```python
from build123d import *

# Parameters (mm, degrees)
RESSALTO_EXTRUS_O1_DEPTH       = 1.9
CONVERTER_S_LIDO1_DEPTH        = 0.7
ARESTA_FLANGE1_STRIP_W         = 8
ARESTA_FLANGE1_STRIP_H         = 1.2
ARESTA_FLANGE1_STRIP_CUT_DEPTH = 532
ARESTA_FLANGE1_DEPTH           = 532
RESSALTO_EXTRUS_O2_DEPTH       = 1.6


# Read off the part's stored shape, not the designer's step: Converter-Sólido1
# Sheet-metal steps are written as plain solids
with BuildPart() as part:
    # Esboço1 → Ressalto-extrusão1 (new body)
    with BuildSketch(Plane.XY):
        with BuildLine():
            Line((-266, -25), (-266, 61))
            Line((-266, 61), (266, 61))
            Line((266, 61), (266, -25))
            Line((266, -25), (208, -25))
            ThreePointArc((208, -25), (199.514718626, -21.485281374), (196, -13))
            Line((196, -13), (196, 0))
            Line((196, 0), (-196, 0))
            Line((-196, 0), (-196, -13))
            ThreePointArc((-196, -13), (-199.514718626, -21.485281374), (-208, -25))
            Line((-208, -25), (-266, -25))
        make_face()
    extrude(amount=RESSALTO_EXTRUS_O1_DEPTH)

    # Converter-Sólido1 outline → Converter-Sólido1 (cut)
    with BuildSketch(Plane.XY):
        with BuildLine():
            Line((-266, -25), (-208, -25))
            ThreePointArc((-208, -25), (-199.514718626, -21.485281374), (-196, -13))
            Line((-196, -13), (-196, 0))
            Line((-196, 0), (196, 0))
            Line((196, 0), (196, -13))
            ThreePointArc((196, -13), (199.514718626, -21.485281374), (208, -25))
            Line((208, -25), (266, -25))
            Line((266, -25), (266, 61))
            Line((266, 61), (-266, 61))
            Line((-266, 61), (-266, -25))
        make_face()
    extrude(amount=CONVERTER_S_LIDO1_DEPTH, mode=Mode.SUBTRACT)

    # Aresta-Flange1 strip (across the edge) → Aresta-Flange1 strip cut (cut)
    with BuildSketch(Plane(origin=(-266, 61, 0.7), x_dir=(0, -1, 0), z_dir=(1, 0, 0))):
        with Locations((-1.2, -0.6)):
            Rectangle(ARESTA_FLANGE1_STRIP_W, ARESTA_FLANGE1_STRIP_H)
    extrude(amount=ARESTA_FLANGE1_STRIP_CUT_DEPTH, mode=Mode.SUBTRACT)

    # Aresta-Flange1 section (across the edge) → Aresta-Flange1 (add)
    with BuildSketch(Plane(origin=(-266, 61, 0.7), x_dir=(0, -1, 0), z_dir=(1, 0, 0))):
        with BuildLine():
            Line((0, 1.6), (0, 24.2))
            Line((0, 24.2), (1.2, 24.2))
            Line((1.2, 24.2), (1.2, 1.6))
            ThreePointArc((1.2, 1.6), (1.66862915, 0.46862915), (2.8, 0))
            Line((2.8, 0), (2.8, -1.2))
            ThreePointArc((2.8, -1.2), (0.820101013, -0.379898987), (0, 1.6))
        make_face()
    extrude(amount=ARESTA_FLANGE1_DEPTH)

    # Esboço5 → Ressalto-extrusão2 (add)
    with BuildSketch(Plane(origin=(266, 0, 0), x_dir=(0, 0, -1), z_dir=(1, 0, 0))):
        Polygon((23.5, 59.8), (-0.7, 35.6), (-0.7, 58.2), (0.9, 59.8), align=None)
    extrude(amount=-RESSALTO_EXTRUS_O2_DEPTH)


solid = part.part
```
Check sheet for the modelled part. Datum: model origin and axes. Units: mm. A direction names the side the tool comes from. Round coordinates to 2 decimals unless told otherwise and drop trailing zeros. Loops run counter-clockwise (first coordinate to the right, second up) from the corner with the lowest first, then second, coordinate; pieces in that order, holes last. Notation, with made-up numbers: M -6.75,82 L 1.25,82 A19 ccw 1.25,108 Z; hole C -4,-20.5 d8. An arc over 180 degrees is marked long. Answer as a JSON object with one key per item and string values.
1. Section check A-A (y = -7). Record the boundary of the cut face in (x, z), plus the area to 3 significant figures.
Reply:
{"outline": "M -266,0.7 L -196,0.7 L -196,1.9 L -266,1.9 Z; M 196,0.7 L 266,0.7 L 266,1.9 L 196,1.9 Z", "area": "168 mm²"}
2. Section check C-C (z = -13.75). Record the boundary of the cut face in (x, y), plus the area to 3 significant figures.
Reply:
{"outline": "M -266,59.8 L 264.4,59.8 L 264.4,50.05 L 266,50.05 L 266,61 L -266,61 Z", "area": "654 mm²"}
3. Scan lines: line 1 (Z direction, x = 117, y = 38); line 2 (Y direction, x = 214, z = -8.75); line 3 (X direction, y = 48, z = -3.25). Record each from-to range of solid material in increasing order.
Reply:
{"line 1": "z = 0.7 to 1.9", "line 2": "y = 59.8 to 61", "line 3": "x = 264.4 to 266"}
4. Section check D-D (y = 25). Record the boundary of the cut face in (x, z), plus the area to 3 significant figures.
Reply:
{"outline": "M -266,0.7 L 266,0.7 L 266,1.9 L -266,1.9 Z", "area": "638 mm²"}
5. Mould release check, pull along X, two halves, no side actions. Record for faces 1 (the flat face through (266, 47, -7)), 2 (the cylindrical face through (199.61, -21.58, 1.29)), 3 (the flat face through (-4, 26, 0.7)), 4 (the flat face through (-266, 18, 1)): pulls with the +X half, pulls with the -X half, needs draft (parallel to the pull), parting line crosses it, or undercut.
Reply:
{"face 1": "pulls with the +X half", "face 2": "undercut", "face 3": "needs draft", "face 4": "pulls with the -X half"}
6. Gauge pin test, flat ends, axial feed: P1, Ø5, axis at x = -44, y = 30, coming from the -Z side; P2, Ø11.5, axis at x = -28, z = -11, coming from the -Y side; P3, Ø7.5, axis at y = 50, z = -13, coming from the -X side. Record the tip position at first contact, or that the pin passes through.
Reply:
{"P1": "stops at z = 0.7", "P2": "stops at y = 59.8", "P3": "stops at x = 264.4"}
7. Access from +Z, -Z, +X, -X, +Y, -Y to the whole of each face (thin tool, end or side, straight path). Record for faces 5 (the cylindrical face through (-199.42, -21.39, 1.29)), 6 (the flat face through (264.4, 53, -6)), 7 (the flat face through (265.2, 47.9, -11.6)).
Reply:
{"face 5": "+Z, -Z, -Y", "face 6": "-Z, -X, -Y", "face 7": "-Z, +X, -X, -Y"}
8. Section check B-B (x = 233). Record the boundary of the cut face in (y, z), plus the area to 3 significant figures.
Reply:
{"outline": "M -25,0.7 L 58.2,0.7 A1.6 cw 59.8,-0.9 L 59.8,-23.5 L 61,-23.5 L 61,-0.9 A2.8 ccw 58.2,1.9 L -25,1.9 Z", "area": "131 mm²"}
